from build123d import *

# Parameters (mm, degrees)
SKETCH_1_W          = 52
SKETCH_1_H          = 52
EXTRUDE_1_DEPTH     = 5
CUT_EXTRUDE_1_DEPTH = 6
CHAMFER_1_SIZE      = 3.5
CHAMFER_2_SIZE      = 0.5
SKETCH_3_W          = 19
SKETCH_3_H          = 40
EXTRUDE_2_DEPTH     = 42
SKETCH_4_W          = 25
SKETCH_4_H          = 52
EXTRUDE_3_DEPTH     = 32
SKETCH_6_W          = 15
SKETCH_6_H          = 35
CUT_EXTRUDE_2_DEPTH = 48
CUT_EXTRUDE_3_REACH = 43.5
SKETCH_7_R          = 9
M3X0_51_D           = 2.5
M3X0_51_DEPTH       = 5.5
M3X0_51_TIP         = 0.751075774
CHAMFER_3_SIZE      = 2
M3X0_52_D           = 2.5
M3X0_52_DEPTH       = 5.5
M3X0_52_TIP         = 0.751075774
SKETCH_13_R         = 3.1
CUT_EXTRUDE_4_DEPTH = 7
CUT_EXTRUDE_5_REACH = 47
SKETCH_14_R         = 1.55
CHAMFER_4_SIZE      = 1
SKETCH_15_W         = 25
SKETCH_15_H         = 32
CUT_EXTRUDE_6_DEPTH = 2.5
SKETCH_16_R         = 6
CUT_EXTRUDE_7_DEPTH = 3
CUT_EXTRUDE_8_REACH = 48.5
SKETCH_17_R         = 5
M3X0_53_D           = 2.5
M3X0_53_DEPTH       = 4.5
M3X0_53_TIP         = 0.751075774
CUT_EXTRUDE_9_REACH = 49
SKETCH_20_R         = 1.5
CHAMFER_5_SIZE      = 0.5


with BuildPart() as part:
    # Эскиз1 → Бобышка-Вытянуть1 (new body)
    with BuildSketch(Plane.XY):
        Rectangle(SKETCH_1_W, SKETCH_1_H)
    extrude(amount=EXTRUDE_1_DEPTH)

    # Эскиз2 → Вырез-Вытянуть1 (cut, through all)
    with BuildSketch(Plane.XY.offset(5)):
        with BuildLine():
            ThreePointArc((-18.5, 21), (-22.767766953, 22.767766953), (-21, 18.5))
            Line((-21, 18.5), (-21, 21))
            Line((-21, 21), (-18.5, 21))
        make_face()
        with BuildLine():
            Line((-21, 21), (-21, 18.5))
            ThreePointArc((-21, 18.5), (-19.232233047, 19.232233047), (-18.5, 21))
            Line((-18.5, 21), (-21, 21))
        make_face()
        with BuildLine():
            ThreePointArc((18.5, 21), (19.232233047, 19.232233047), (21, 18.5))
            Line((21, 18.5), (21, 21))
            Line((21, 21), (18.5, 21))
        make_face()
        with BuildLine():
            Line((21, 21), (21, 18.5))
            ThreePointArc((21, 18.5), (22.767766953, 19.232233047), (23.5, 21))
            ThreePointArc((23.5, 21), (21, 23.5), (18.5, 21))
            Line((18.5, 21), (21, 21))
        make_face()
        with BuildLine():
            Line((-21, -18.5), (-21, -21))
            Line((-21, -21), (-18.5, -21))
            ThreePointArc((-18.5, -21), (-19.232233047, -19.232233047), (-21, -18.5))
        make_face()
        with BuildLine():
            Line((-18.5, -21), (-21, -21))
            Line((-21, -21), (-21, -18.5))
            ThreePointArc((-21, -18.5), (-22.767766953, -22.767766953), (-18.5, -21))
        make_face()
        with BuildLine():
            ThreePointArc((21, -18.5), (19.232233047, -19.232233047), (18.5, -21))
            Line((18.5, -21), (21, -21))
            Line((21, -21), (21, -18.5))
        make_face()
        with BuildLine():
            Line((21, -21), (18.5, -21))
            ThreePointArc((18.5, -21), (21, -23.5), (23.5, -21))
            ThreePointArc((23.5, -21), (22.767766953, -19.232233047), (21, -18.5))
            Line((21, -18.5), (21, -21))
        make_face()
    extrude(amount=-CUT_EXTRUDE_1_DEPTH, mode=Mode.SUBTRACT)

    # Фаска1
    chamfer_1_edges = [part.edges().sort_by_distance(p)[0] for p in [
        (26, -26, 2.5),
        (-26, -26, 2.5),
        (-26, 26, 2.5),
        (26, 26, 2.5),
    ]]
    chamfer(chamfer_1_edges, length=CHAMFER_1_SIZE)

    # Фаска2
    chamfer_2_edges = [part.edges().sort_by_distance(p)[0] for p in [
        (23.5, 21, 5),
        (-21, 23.5, 5),
        (-23.5, -21, 5),
        (18.5, -21, 5),
    ]]
    chamfer(chamfer_2_edges, length=CHAMFER_2_SIZE)

    # Эскиз3 → Бобышка-Вытянуть2 (add)
    with BuildSketch(Plane.XY.offset(5)):
        Rectangle(SKETCH_3_W, SKETCH_3_H)
    extrude(amount=EXTRUDE_2_DEPTH)

    # Эскиз4 → Бобышка-Вытянуть3 (add)
    with BuildSketch(Plane.XY.offset(47)):
        with Locations((-3, 0)):
            Rectangle(SKETCH_4_W, SKETCH_4_H)
    extrude(amount=-EXTRUDE_3_DEPTH)

    # Эскиз6 → Вырез-Вытянуть2 (cut, through all)
    with BuildSketch(Plane.XY.offset(47)):
        Rectangle(SKETCH_6_W, SKETCH_6_H)
    extrude(amount=-CUT_EXTRUDE_2_DEPTH, mode=Mode.SUBTRACT)

    # Эскиз7 → Вырез-Вытянуть3 (cut, up to next)
    with BuildSketch(Plane.ZY.offset(15.5), mode=Mode.PRIVATE) as cut_extrude_3_sk1:
        with Locations((30, 0)):
            Circle(SKETCH_7_R)
    cut_extrude_3_tool1 = extrude(cut_extrude_3_sk1.sketch, amount=-CUT_EXTRUDE_3_REACH, mode=Mode.PRIVATE) & part.part
    add(cut_extrude_3_tool1.solids().sort_by_distance((-15.5, 0, 30))[0], mode=Mode.SUBTRACT)

    # Отверстие обработанное метчиком M3x0.51
    with Locations(Plane(origin=(-15.5, 11, 39), x_dir=(0, 0, -1), z_dir=(-1, 0, 0))):
        with Locations((0, 0), (0, 22), (18, 22), (18, 0)):
            Hole(M3X0_51_D / 2, depth=M3X0_51_DEPTH)
            with Locations((0, 0, -(M3X0_51_DEPTH + M3X0_51_TIP / 2))):  # 118° drill point
                Cone(0, M3X0_51_D / 2, M3X0_51_TIP, mode=Mode.SUBTRACT)

    # Фаска3
    chamfer_3_edges = [part.edges().sort_by_distance(p)[0] for p in [
        (9.5, 26, 31),
        (9.5, -26, 31),
        (-15.5, -26, 31),
        (-15.5, 26, 31),
    ]]
    chamfer(chamfer_3_edges, length=CHAMFER_3_SIZE)

    # Отверстие обработанное метчиком M3x0.52
    with Locations(Plane(origin=(5.5, 20, 47), x_dir=(1, 0, 0), z_dir=(0, 0, 1))):
        with Locations((0, 0), (-17, -20), (0, -40)):
            Hole(M3X0_52_D / 2, depth=M3X0_52_DEPTH)
            with Locations((0, 0, -(M3X0_52_DEPTH + M3X0_52_TIP / 2))):  # 118° drill point
                Cone(0, M3X0_52_D / 2, M3X0_52_TIP, mode=Mode.SUBTRACT)

    # Эскиз13 → Вырез-Вытянуть4 (cut)
    with BuildSketch(Plane(origin=(0, -26, 0), x_dir=(-1, 0, 0), z_dir=(0, -1, 0))):
        with Locations((1, -30)):
            Circle(SKETCH_13_R)
    extrude(amount=-CUT_EXTRUDE_4_DEPTH, mode=Mode.SUBTRACT)

    # Эскиз14 → Вырез-Вытянуть5 (cut, up to next)
    with BuildSketch(Plane.XZ.offset(19), mode=Mode.PRIVATE) as cut_extrude_5_sk1:
        with Locations((-1, 30)):
            Circle(SKETCH_14_R)
    cut_extrude_5_tool1 = extrude(cut_extrude_5_sk1.sketch, amount=-CUT_EXTRUDE_5_REACH, mode=Mode.PRIVATE) & part.part
    add(cut_extrude_5_tool1.solids().sort_by_distance((-1, -19, 30))[0], mode=Mode.SUBTRACT)

    # Фаска4
    chamfer_4_edges = [part.edges().sort_by_distance(p)[0] for p in [
        (2.1, -26, 30),
    ]]
    chamfer(chamfer_4_edges, length=CHAMFER_4_SIZE)

    # Эскиз15 → Вырез-Вытянуть6 (cut)
    with BuildSketch(Plane(origin=(0, 26, 0), x_dir=(1, 0, 0), z_dir=(0, 1, 0))):
        with Locations((-3, -31)):
            Rectangle(SKETCH_15_W, SKETCH_15_H)
    extrude(amount=-CUT_EXTRUDE_6_DEPTH, mode=Mode.SUBTRACT)

    # Эскиз16 → Вырез-Вытянуть7 (cut)
    with BuildSketch(Plane(origin=(0, 23.5, 0), x_dir=(1, 0, 0), z_dir=(0, 1, 0))):
        with Locations((-1, -30)):
            Circle(SKETCH_16_R)
    extrude(amount=-CUT_EXTRUDE_7_DEPTH, mode=Mode.SUBTRACT)

    # Эскиз17 → Вырез-Вытянуть8 (cut, up to next)
    with BuildSketch(Plane(origin=(0, 20.5, 0), x_dir=(1, 0, 0), z_dir=(0, 1, 0)), mode=Mode.PRIVATE) as cut_extrude_8_sk1:
        with Locations((-1, -30)):
            Circle(SKETCH_17_R)
    cut_extrude_8_tool1 = extrude(cut_extrude_8_sk1.sketch, amount=-CUT_EXTRUDE_8_REACH, mode=Mode.PRIVATE) & part.part
    add(cut_extrude_8_tool1.solids().sort_by_distance((-1, 20.5, 30))[0], mode=Mode.SUBTRACT)

    # Отверстие обработанное метчиком M3x0.53
    with Locations(Plane(origin=(-1, 23.5, 40.5), x_dir=(0, 0, 1), z_dir=(0, 1, 0))):
        with Locations((0, 0), (-21, 0)):
            Hole(M3X0_53_D / 2, depth=M3X0_53_DEPTH)
            with Locations((0, 0, -(M3X0_53_DEPTH + M3X0_53_TIP / 2))):  # 118° drill point
                Cone(0, M3X0_53_D / 2, M3X0_53_TIP, mode=Mode.SUBTRACT)

    # Эскиз20 → Вырез-Вытянуть9 (cut, up to next)
    with BuildSketch(Plane(origin=(0, 0, 0), x_dir=(-1, 0, 0), z_dir=(0, 0, -1)), mode=Mode.PRIVATE) as cut_extrude_9_sk1:
        with Locations((-17, 0)):
            Circle(SKETCH_20_R)
    cut_extrude_9_tool1 = extrude(cut_extrude_9_sk1.sketch, amount=-CUT_EXTRUDE_9_REACH, mode=Mode.PRIVATE) & part.part
    add(cut_extrude_9_tool1.solids().sort_by_distance((17, 0, 0))[0], mode=Mode.SUBTRACT)
    # Эскиз20 → Вырез-Вытянуть9 (cut, up to next)
    with BuildSketch(Plane(origin=(0, 0, 0), x_dir=(-1, 0, 0), z_dir=(0, 0, -1)), mode=Mode.PRIVATE) as cut_extrude_9_sk2:
        with Locations((17, 0)):
            Circle(SKETCH_20_R)
    cut_extrude_9_tool2 = extrude(cut_extrude_9_sk2.sketch, amount=-CUT_EXTRUDE_9_REACH, mode=Mode.PRIVATE) & part.part
    add(cut_extrude_9_tool2.solids().sort_by_distance((-17, 0, 0))[0], mode=Mode.SUBTRACT)

    # Фаска5
    chamfer_5_edges = [part.edges().sort_by_distance(p)[0] for p in [
        (18.5, 0, 5),
        (-15.5, 0, 5),
    ]]
    chamfer(chamfer_5_edges, length=CHAMFER_5_SIZE)


solid = part.part
Design review of the part built by this model. Coordinates are the model's own, in mm. A direction names the side the tool comes from. Give positions to 0.01 mm unless a question says otherwise; leave off trailing zeros. Loops run counter-clockwise (first coordinate to the right, second up) from the corner with the lowest first, then second, coordinate; pieces in that order, holes last. Notation, with made-up numbers: (6.25, -26.5) -> (53.25, -26.5) arc R25 cw to (53.25, 11.5) -> close; hole circle Ø9 at (27.25, 85.25). An arc over 180 degrees is marked (long way). One line per question, with ' | ' between items. Start each with the question number.
(1) For faces 5 (the face through (5.77, 18.78, 44.21)), 6 (the face through (-6, 23.5, 34)), 7 (the face through (-12, -1, 15)), 8 (the face through (-2.3, -19, 31.3)), list the 3-axis set-ups (+Z, -Z, +X, -X, +Y, -Y) from which the entire face can be reached by the end or side of a thin tool; tool diameter is ignored.
(2) Draft analysis for pull direction X (two halves, no side actions). For faces 1 (the face through (-9.5, 0, 10)), 2 (the face through (0, -26, 2)), 3 (the face through (-1.202, -18.26, 31.537)), 4 (the face through (-1.479, 21.218, 18.345)), state which applies: +X half, -X half, draft (parallel to the pull), parting line (faces both ways), or undercut.
(3) Insertion check: P1, Ø4, axis at x = -1, z = 30, coming from the +Y side; P2, Ø6, axis at x = 19.5, y = -16, coming from the +Z side; P3, Ø4, axis at y = 13, z = 29.5, coming from the +X side; P4, Ø3, axis at x = -21, y = 21, coming from the -Z side. Each pin has a flat end and moves straight along its axis. Give the tip position at first contact, or say it passes through.
(4) We need section A-A (z = 8.5). State the section outline as (x, y) points, and give its area (3 significant figures).
(5) For line 1 (X direction, y = 0, z = 42.6); line 2 (Z direction, x = -1, y = 19.6); line 3 (X direction, y = -9, z = 22.5), list the stretches that pass through material, from the lowest coordinate up.
(6) We need section B-B (y = 6). State the section outline as (x, z) points, and give its area (3 significant figures).
The answers:
1) face 5: +Z | face 6: +Z, +X, -X, +Y | face 7: -X | face 8: -Y
2) face 1: -X half | face 2: draft | face 3: undercut | face 4: undercut
3) P1: stops at y = -17.5 | P2: stops at z = 5 | P3: stops at x = 9.5 | P4: passes through
4) outline: (-9.5, -20) -> (9.5, -20) -> (9.5, 20) -> (-9.5, 20) -> close; hole (-7.5, -17.5) -> (7.5, -17.5) -> (7.5, 17.5) -> (-7.5, 17.5) -> close | area: 235 mm^2
5) line 1: x = -15.5 to -12.75, -10.25 to -7.5, 7.5 to 9.5 | line 2: z = 0 to 18.25, 20.75 to 25, 35 to 39.25, 41.75 to 47 | line 3: x = -15.5 to -7.5, 7.5 to 9.5
6) outline: (-26, 0) -> (-7.5, 0) -> (-7.5, 23.29) -> (-15.5, 23.29) -> (-15.5, 15) -> (-9.5, 15) -> (-9.5, 5) -> (-26, 5) -> close; (-15.5, 36.71) -> (-7.5, 36.71) -> (-7.5, 47) -> (-15.5, 47) -> close; (7.5, 0) -> (26, 0) -> (26, 5) -> (9.5, 5) -> (9.5, 47) -> (7.5, 47) -> close | area: 438 mm^2
